Model file for the job. Use its own axes, mm. A direction names the side the tool comes from. Give positions to 0.01 mm unless a question says otherwise; leave off trailing zeros. Write each loop counter-clockwise with the first axis right and the second up, starting at its lowest first coordinate (ties: lowest second). Pieces come first, ordered by that corner, then holes.
```python
from build123d import *

# Parameters (mm, degrees)
SKETCH2_R          = 2
CUT_EXTRUDE1_DEPTH = 4


with BuildPart() as part:
    # Sketch1 → Revolve1 (revolve)
    with BuildSketch(Plane(origin=(0, 0, 0), x_dir=(0, 0, -1), z_dir=(1, 0, 0))):
        with BuildLine():
            Line((-7.15, 3.5), (-4.15, 3.5))
            Line((-4.15, 3.5), (-4.15, 0))
            Line((-4.15, 0), (0, 0))
            Line((0, 0), (0, -41))
            Line((0, -41), (-17.15, -41))
            Line((-17.15, -41), (-17.15, -37))
            Line((-17.15, -37), (-9.15, -37))
            ThreePointArc((-9.15, -37), (-7.735786438, -36.414213562), (-7.15, -35))
            Line((-7.15, -35), (-7.15, 3.5))
        make_face()
    revolve(axis=Axis((0, 0, 0), (0, -1, 0)))

    # Sketch2 → Cut-Extrude1 (cut)
    with BuildSketch(Plane(origin=(0, -37, 0), x_dir=(1, 0, 0), z_dir=(0, 1, 0))):
        with Locations(Location((0, 12.15, 0), (0, 0, 270))):
            Circle(SKETCH2_R)
        with Locations(Location((12.15, 0, 0), (0, 0, 270))):
            Circle(SKETCH2_R)
        with Locations(Location((0, -12.15, 0), (0, 0, 270))):
            Circle(SKETCH2_R)
        with Locations(Location((-12.15, 0, 0), (0, 0, 270))):
            Circle(SKETCH2_R)
    extrude(amount=-CUT_EXTRUDE1_DEPTH, mode=Mode.SUBTRACT)


solid = part.part
```
1. Slice it at B-B, the plane x = 13.5. Write the cut outline in (y, z).
Calculated:
outline: (-41, -10.58) - (-37, -10.58) - (-37, -1.48) - (-41, -1.48) - close; (-41, 1.48) - (-37, 1.48) - (-37, 10.58) - (-41, 10.58) - close
2. Pin check, flat tips, straight feed: P1, Ø6, axis at x = -8, z = -9.5, coming from the +Y side; P2, Ø6, axis at x = 6, y = -23, coming from the +Z side; P3, Ø10, axis at x = -10, y = -29, coming from the -Z side. Stop position of each tip, or through.
Calculated:
P1: stops at y = -37
P2: stops at z = 6.49
P3: stops at z = -5.11
3. Pull direction Z, two halves, no side cores. Call faces 1 (the cylindrical face through (0.088, -38.972, -14.148)), 2 (the flat face through (3.1, 3.5, 3.1)), 3 (the cylindrical face through (-5.15, -38.97, 16.36)), 4 (the cylindrical face through (-10.167, -38.972, -0.26)): +Z half, -Z half, draft (parallel to the pull), parting line (faces both ways), or undercut.
Calculated:
face 1: undercut
face 2: draft
face 3: parting line
face 4: undercut
4. Which spindle directions (+Z, -Z, +X, -X, +Y, -Y) get a long thin tool onto all of the face, cutting with end or side? Do faces 5 (the flat face through (0, -41, 0)), 6 (the cylindrical face through (-7.09, -15.48, -0.93)). Say none if no direction does.
Calculated:
face 5: +Z, -Z, +X, -X, -Y
face 6: +Y
5. Slice it at C-C, the plane z = -12.15. Write the cut outline in (x, y).
Calculated:
outline: (-12.1, -41) - (-2, -41) - (-2, -37) - (-12.1, -37) - close; (2, -41) - (12.1, -41) - (12.1, -37) - (2, -37) - close
6. Slice it at D-D, the plane y = -29. Write the cut outline in (x, z).
Calculated:
outline: circle Ø14.3 at (0, 0)
7. Slice it at A-A, the plane z = 0. Write the cut outline in (x, y), and give its area (3 significant figures).
Calculated:
outline: (-17.15, -41) - (-14.15, -41) - (-14.15, -37) - (-17.15, -37) - close; (-10.15, -41) - (10.15, -41) - (10.15, -37) - (9.15, -37) arc R2 cw to (7.15, -35) - (7.15, 3.5) - (4.15, 3.5) - (4.15, 0) - (-4.15, 0) - (-4.15, 3.5) - (-7.15, 3.5) - (-7.15, -35) arc R2 cw to (-9.15, -37) - (-10.15, -37) - close; (14.15, -41) - (17.15, -41) - (17.15, -37) - (14.15, -37) - close
area: 657 mm2
8. Probe probe 1 along X at (y, z) = (-37.9, 0); probe 2 along Y at (x, z) = (0, -3); probe 3 along Y at (x, z) = (13.5, -2.5). List the from-to ranges inside material, lowest first.
Calculated:
probe 1: x = -17.15 to -14.15, -10.15 to 10.15, 14.15 to 17.15
probe 2: y = -41 to 0
probe 3: y = -41 to -37
